```python
from build123d import *

# Parameters (mm, degrees)
SKETCH1_R           = 4.75
BOSS_EXTRUDE1_DEPTH = 4.5
SKETCH2_R           = 7
BOSS_EXTRUDE2_DEPTH = 1
SKETCH3_W           = 3
SKETCH3_H           = 3
CUT_EXTRUDE1_DEPTH  = 12.324751653
FILLET3_R           = 0.5
SKETCH4_W           = 5.2
SKETCH4_H           = 2.5
CUT_EXTRUDE2_DEPTH  = 12.324751763


with BuildPart() as part:
    # Sketch1 → Boss-Extrude1 (new body)
    with BuildSketch(Plane(origin=(0, 0, 0), x_dir=(1, 0, 0), z_dir=(0, 1, 0))):
        with Locations(Location((0, 0, 0), (0, 0, 270))):
            Circle(SKETCH1_R)
    extrude(amount=BOSS_EXTRUDE1_DEPTH)

    # Sketch2 → Boss-Extrude2 (add)
    with BuildSketch(Plane(origin=(0, 4.5, 0), x_dir=(1, 0, 0), z_dir=(0, 1, 0))):
        with Locations(Location((0, 0, 0), (0, 0, 270))):
            Circle(SKETCH2_R)
    extrude(amount=BOSS_EXTRUDE2_DEPTH)

    # Sketch3 → Cut-Extrude1 (cut, through all)
    with BuildSketch(Plane(origin=(0, 5.5, 0), x_dir=(1, 0, 0), z_dir=(0, 1, 0))):
        with Locations((0, 3.443002763)):
            Rectangle(SKETCH3_W, SKETCH3_H)
        with Locations((0, -3.443002763)):
            Rectangle(SKETCH3_W, SKETCH3_H)
    extrude(amount=-CUT_EXTRUDE1_DEPTH, mode=Mode.SUBTRACT)

    # Fillet3
    fillet3_edges = [part.edges().sort_by_distance(p)[0] for p in [
        (-4.75, 0, 0),
        (4.75, 0, 0),
        (0, 4.5, -7),
        (0, 5.5, -7),
    ]]
    fillet(fillet3_edges, radius=FILLET3_R - 0.0001)  # a hair under: the kernel refuses the full size

    # Sketch4 → Cut-Extrude2 (cut, through all)
    with BuildSketch(Plane(origin=(0, 5.5, 0), x_dir=(1, 0, 0), z_dir=(0, 1, 0))):
        Rectangle(SKETCH4_W, SKETCH4_H)
    extrude(amount=-CUT_EXTRUDE2_DEPTH, mode=Mode.SUBTRACT)


solid = part.part
```
Geometry check sheet. Reference: the model listing, model coordinates, mm. A direction names the side the tool comes from. Coordinates: 2 decimals unless noted, no trailing zeros. Write each loop counter-clockwise with the first axis right and the second up, starting at its lowest first coordinate (ties: lowest second). Pieces come first, ordered by that corner, then holes. Notation, with made-up numbers: M 47,-14.5 L 95,-14.5 A24 cw 95,9.5 Z; hole C 41.25,4 d10. An arc over 180 degrees is marked long. Use one line per item in the form item = value. Start each with the question number.
1) Thickness scan on probe 1 along Z at (x, y) = (-0.25, 2.6); probe 2 along X at (y, z) = (0.4, -2.75); probe 3 along X at (y, z) = (1, -3.75). Record the ranges inside material, lowest first. Write a range as from..to.
2) Section check A-A on y = 4.1. Enter the section's corners in (x, z), and give its area (3 significant figures).
3) Set-up check for faces 1 (the flat face through (-1.5, 3, -3)), 2 (the flat face through (0.1, 5.5, -1.5)): record each of +Z, -Z, +X, -X, +Y, -Y from which the full face is reachable in a straight line by a thin tool's end or side.
4) Go/stop test with flat-tipped pins: pin 1 Ø1.5 at (y, z) = (1.5, -3.5) entering from +X; pin 2 Ø6 at (x, z) = (-0.5, 3) entering from -Y; pin 3 Ø1.5 at (x, y) = (0, 2) entering from -Z; pin 4 Ø3 at (y, z) = (1, -2.5) entering from -X. Record where each tip stops, or that it passes through.
5) Release check for a two-part mould opening along X. For faces 3 (the flat face through (0, 5, -4.943)), 4 (the cylindrical face through (4.75, 2.47, 0.08)), 5 (the cylindrical face through (-4.75, 2.47, -0.08)), 6 (the flat face through (-5, 4.5, 0)) record: pulls with the +X half, pulls with the -X half, needs draft (parallel to the pull), parting line crosses it, or undercut.
6) Section check B-B on x = 0. State how many separate pieces and enclosed holes the cut face has, and give its area (3 significant figures).
Responses:
q1.probe_1 = -1.94..-1.25, 1.25..1.94
q1.probe_2 = -3.86..-1.5, 1.5..3.86
q1.probe_3 = -2.92..-1.5, 1.5..2.92
q2.outline = M -1.5,-4.51 L -1.5,-1.94 L 1.5,-1.94 L 1.5,-4.51 A4.75 ccw 1.5,4.51 L 1.5,1.94 L -1.5,1.94 L -1.5,4.51 A4.75 ccw Z; hole M -2.6,-1.25 L 2.6,-1.25 L 2.6,1.25 L -2.6,1.25 Z
q2.area = 41.5 mm2
q3.face_1 = +Y, -Y
q3.face_2 = +Z, -Z, +X, -X, +Y
q4.pin_1 = 3.87
q4.pin_2 = 0
q4.pin_3 = -1.94
q4.pin_4 = -4.64
q5.face_3 = undercut
q5.face_4 = pulls with the +X half
q5.face_5 = pulls with the -X half
q5.face_6 = needs draft
q6.separate_pieces = 4
q6.enclosed_holes = 0
q6.area = 11.5 mm2
